from build123d import *

# Parameters (mm, degrees)
SKETCH1_W           = 150
SKETCH1_H           = 200
BOSS_EXTRUDE1_DEPTH = 5
SKETCH2_W           = 150
SKETCH2_H           = 200
SKETCH2_W_2         = 145
SKETCH2_H_2         = 195
BOSS_EXTRUDE2_DEPTH = 100
SKETCH3_R           = 3.175
CUT_EXTRUDE1_DEPTH  = 50
SKETCH4_R           = 4
SKETCH4_R_2         = 3.175
BOSS_EXTRUDE3_DEPTH = 2
SKETCH5_R           = 3.175
CUT_EXTRUDE2_DEPTH  = 14
SKETCH6_R           = 4
SKETCH6_R_2         = 3.175
BOSS_EXTRUDE4_DEPTH = 2
SKETCH7_R           = 3.174999996
SKETCH7_R_2         = 3.175
CUT_EXTRUDE3_DEPTH  = 10


with BuildPart() as part:
    # Sketch1 → Boss-Extrude1 (new body)
    with BuildSketch(Plane(origin=(0, 0, 0), x_dir=(1, 0, 0), z_dir=(0, 1, 0))):
        Rectangle(SKETCH1_W, SKETCH1_H)
    extrude(amount=BOSS_EXTRUDE1_DEPTH)

    # Sketch2 → Boss-Extrude2 (add)
    with BuildSketch(Plane(origin=(0, 5, 0), x_dir=(1, 0, 0), z_dir=(0, 1, 0))):
        Rectangle(SKETCH2_W, SKETCH2_H)
        Rectangle(SKETCH2_W_2, SKETCH2_H_2, mode=Mode.SUBTRACT)
    extrude(amount=BOSS_EXTRUDE2_DEPTH)

    # Sketch3 → Cut-Extrude1 (cut)
    with BuildSketch(Plane.XY.offset(100)):
        with Locations((0, 90)):
            Circle(SKETCH3_R)
    extrude(amount=-CUT_EXTRUDE1_DEPTH, mode=Mode.SUBTRACT)

    # Sketch4 → Boss-Extrude3 (add)
    with BuildSketch(Plane.XY.offset(100)):
        with Locations((0, 90)):
            Circle(SKETCH4_R)
        with Locations((0, 90)):
            Circle(SKETCH4_R_2, mode=Mode.SUBTRACT)
    extrude(amount=BOSS_EXTRUDE3_DEPTH)

    # Sketch5 → Cut-Extrude2 (cut)
    with BuildSketch(Plane(origin=(0, 0, -100), x_dir=(-1, 0, 0), z_dir=(0, 0, -1))):
        with Locations((0, 10)):
            Circle(SKETCH5_R)
    extrude(amount=-CUT_EXTRUDE2_DEPTH, mode=Mode.SUBTRACT)

    # Sketch6 → Boss-Extrude4 (add)
    with BuildSketch(Plane(origin=(0, 0, -100), x_dir=(-1, 0, 0), z_dir=(0, 0, -1))):
        with Locations((0, 10)):
            Circle(SKETCH6_R)
        with Locations((0, 10)):
            Circle(SKETCH6_R_2, mode=Mode.SUBTRACT)
    extrude(amount=BOSS_EXTRUDE4_DEPTH)

    # Sketch7 → Cut-Extrude3 (cut)
    with BuildSketch(Plane.ZY.offset(75)):
        with Locations((-60, 15)):
            Circle(SKETCH7_R)
        with Locations((60, 85)):
            Circle(SKETCH7_R_2)
    extrude(amount=-CUT_EXTRUDE3_DEPTH, mode=Mode.SUBTRACT)


solid = part.part
The model under review builds one solid part; all positions refer to its coordinate system, in mm. A direction names the side the tool comes from. Coordinates: 2 decimals unless noted, no trailing zeros. Write each loop counter-clockwise with the first axis right and the second up, starting at its lowest first coordinate (ties: lowest second). Pieces come first, ordered by that corner, then holes. Notation, with made-up numbers: (71.25, 86.25) - (111.25, 86.25) arc R23 ccw to (111.25, 101.25) - close; hole circle Ø6 at (63, 65). An arc over 180 degrees is marked (long way). Answer as CSV lines item,"result".
(1) We need section D-D (x = 41). Give the boundary of the cut face in (y, z), plus the area to 3 significant figures.
Data:
outline,"(0, -100) - (105, -100) - (105, -97.5) - (5, -97.5) - (5, 97.5) - (105, 97.5) - (105, 100) - (0, 100) - close"
area,"1,500 mm2"
(2) Clearance check with flat-ended pins moving along their axes: pin 1 Ø12 at (x, z) = (47.5, -34.5) entering from +Y; pin 2 Ø12 at (x, y) = (54, 45.5) entering from -Z; pin 3 Ø10 at (x, y) = (0, 10) entering from +Z. State where each tip first meets the part, or that it passes through.
Data:
pin 1,"stops at y = 5"
pin 2,"stops at z = -100"
pin 3,"stops at z = 100"
(3) Mouldability with a two-part tool opening along Y and no side actions: class faces 1 (the cylindrical face through (-73.768, 87.677, 61.707)), 2 (the flat face through (-75, 52, 1)), 3 (the flat face through (-1, 0, -1)), 4 (the cylindrical face through (0.521, 13.966, -100.986)) as pulls with the +Y half, pulls with the -Y half, needs draft (parallel to the pull), parting line crosses it, or undercut.
Data:
face 1,"undercut"
face 2,"needs draft"
face 3,"pulls with the -Y half"
face 4,"parting line crosses it"
(4) We need section C-C (z = 60). Give the boundary of the cut face in (x, y) (3 decimals), plus the area to 3 significant figures.
Data:
outline,"(-75, 0) - (75, 0) - (75, 105) - (72.5, 105) - (72.5, 5) - (-72.5, 5) - (-72.5, 81.825) - (-75, 81.825) - close; (-75, 88.175) - (-72.5, 88.175) - (-72.5, 105) - (-75, 105) - close"
area,"1,230 mm2"
(5) We need section B-B (y = 40). Give the boundary of the cut face in (x, z), plus the area to 4 significant figures.
Data:
outline,"(-75, -100) - (75, -100) - (75, 100) - (-75, 100) - close; hole (-72.5, -97.5) - (72.5, -97.5) - (72.5, 97.5) - (-72.5, 97.5) - close"
area,"1,725 mm2"
(6) For line 1 along Z through (x, y) = (45.5, 19.5); line 2 along Y through (x, z) = (-73, -60) (3 decimals); line 3 along Y through (x, z) = (-73.95, 60) (3 decimals), list the stretches that pass through material, from the lowest coordinate up. Write a range as [from, to].
Data:
line 1,"z = [-100, -97.5], [97.5, 100]"
line 2,"y = [0, 11.825], [18.175, 105]"
line 3,"y = [0, 81.825], [88.175, 105]"
(7) Tool access review of faces 5 (the cylindrical face through (1.846, 86.451, 100.986)), 6 (the cylindrical face through (-73.77, 15.14, -63.17)), 7 (the flat face through (-72.5, 54, 1)): name each direction out of +Z, -Z, +X, -X, +Y, -Y from which nothing blocks a thin tool from reaching the whole face with its end or side.
Data:
face 5,"+Z"
face 6,"-X"
face 7,"+Y"
(8) We need section A-A (x = 0). Give the boundary of the cut face in (y, z) (3 decimals), plus the area to 3 significant figures.
Data:
outline,"(0, -100) - (6, -100) - (6, -102) - (6.825, -102) - (6.825, -97.5) - (5, -97.5) - (5, 97.5) - (86.825, 97.5) - (86.825, 102) - (86, 102) - (86, 100) - (0, 100) - close; (13.175, -102) - (14, -102) - (14, -100) - (105, -100) - (105, -97.5) - (13.175, -97.5) - close; (93.175, 97.5) - (105, 97.5) - (105, 100) - (94, 100) - (94, 102) - (93.175, 102) - close"
area,"1,470 mm2"
